from build123d import *

# Parameters (mm, degrees)
BOSS_EXTRUDE1_DEPTH             = 12.7
BOSS_EXTRUDE4_REACH             = 14.7
BOSS_EXTRUDE4_DIRECTION_2_REACH = 14.7
SKETCH6_W                       = 16.51
SKETCH6_H                       = 15.748
CUT_EXTRUDE2_DEPTH              = 53.07
SKETCH11_W                      = 11.43
SKETCH11_H                      = 7.62
CUT_EXTRUDE3_DEPTH              = 3.81
SKETCH15_R                      = 3.2385
CUT_EXTRUDE4_DEPTH              = 25.4


with BuildPart() as part:
    # Sketch1 → Boss-Extrude1 (new body, symmetric)
    with BuildSketch(Plane.XY):
        with BuildLine():
            Line((-20.32, 16.002), (-20.32, -25.4))
            Line((-20.32, -25.4), (20.32, -25.4))
            Line((20.32, -25.4), (20.32, 16.002))
            Line((20.32, 16.002), (2.794, 16.002))
            Line((2.794, 16.002), (2.794, 28.1305))
            Line((2.794, 28.1305), (6.477, 28.1305))
            ThreePointArc((6.477, 28.1305), (6.946330803, 28.444096816), (6.836210245, 28.997710245))
            Line((6.836210245, 28.997710245), (3.706459265, 32.127461224))
            ThreePointArc((3.706459265, 32.127461224), (2.882423959, 32.678064013), (1.910408041, 32.87141))
            Line((1.910408041, 32.87141), (-1.910408041, 32.87141))
            ThreePointArc((-1.910408041, 32.87141), (-2.882423959, 32.678064013), (-3.706459265, 32.127461224))
            Line((-3.706459265, 32.127461224), (-6.836210245, 28.997710245))
            ThreePointArc((-6.836210245, 28.997710245), (-6.946330803, 28.444096816), (-6.477, 28.1305))
            Line((-6.477, 28.1305), (-2.794, 28.1305))
            Line((-2.794, 28.1305), (-2.794, 16.002))
            Line((-2.794, 16.002), (-20.32, 16.002))
        make_face()
        Polygon((-4.106115114, 7.112), (-8.212230229, 0), (-4.106115114, -7.112), (4.106115114, -7.112), (8.212230229, 0), (4.106115114, 7.112), align=None, mode=Mode.SUBTRACT)
    extrude(amount=BOSS_EXTRUDE1_DEPTH, both=True)

    # Boss-Extrude4: up to this face of the body (flat: up to its plane)
    boss_extrude4_end = Plane(part.part.faces().sort_by_distance((-6.289975232, 28.715968196, 12.7))[0])
    # Sketch10 → Boss-Extrude4 (add, up to the picked face)
    with BuildSketch(Plane.XY, mode=Mode.PRIVATE) as boss_extrude4_sk1:
        Polygon((-20.32, -25.4), (-20.32, -46.99), (-31.75, -46.99), (-31.75, -50.8), (-16.51, -50.8), (-16.51, -25.4), align=None)
    boss_extrude4_tool1 = split(extrude(boss_extrude4_sk1.sketch, amount=BOSS_EXTRUDE4_REACH, mode=Mode.PRIVATE), bisect_by=boss_extrude4_end, keep=Keep.BOTH, mode=Mode.PRIVATE)
    add(boss_extrude4_tool1.solids().sort_by_distance((-20.023788, -36.195, 0))[0])

    # Boss-Extrude4 direction 2: up to this face of the body (flat: up to its plane)
    boss_extrude4_direction_2_end = Plane(part.part.faces().sort_by_distance((-6.289975232, 28.715968196, -12.7))[0])
    # Sketch10 → Boss-Extrude4 direction 2 (add, up to the picked face)
    with BuildSketch(Plane.XY, mode=Mode.PRIVATE) as boss_extrude4_direction_2_sk1:
        Polygon((-20.32, -25.4), (-20.32, -46.99), (-31.75, -46.99), (-31.75, -50.8), (-16.51, -50.8), (-16.51, -25.4), align=None)
    boss_extrude4_direction_2_tool1 = split(extrude(boss_extrude4_direction_2_sk1.sketch, amount=-BOSS_EXTRUDE4_DIRECTION_2_REACH, mode=Mode.PRIVATE), bisect_by=boss_extrude4_direction_2_end, keep=Keep.BOTH, mode=Mode.PRIVATE)
    add(boss_extrude4_direction_2_tool1.solids().sort_by_distance((-20.023788, -36.195, 0))[0])

    # Sketch6 → Cut-Extrude2 (cut, through all)
    with BuildSketch(Plane(origin=(20.32, 0, 0), x_dir=(0, 0, -1), z_dir=(1, 0, 0))):
        with Locations((0, -17.526)):
            Rectangle(SKETCH6_W, SKETCH6_H)
    extrude(amount=-CUT_EXTRUDE2_DEPTH, mode=Mode.SUBTRACT)

    # Sketch11 → Cut-Extrude3 (cut)
    with BuildSketch(Plane(origin=(0, -46.99, 0), x_dir=(1, 0, 0), z_dir=(0, 1, 0))):
        with Locations((-26.035, 0)):
            Rectangle(SKETCH11_W, SKETCH11_H)
    extrude(amount=-CUT_EXTRUDE3_DEPTH, mode=Mode.SUBTRACT)

    # Sketch15 → Cut-Extrude4 (cut)
    with BuildSketch(Plane.XY.offset(12.7)):
        with Locations((0, -19.05)):
            Circle(SKETCH15_R)
    extrude(amount=-CUT_EXTRUDE4_DEPTH, mode=Mode.SUBTRACT)


solid = part.part
Design review of the part built by this model. Coordinates are the model's own, in mm. A direction names the side the tool comes from. Round coordinates to 2 decimals unless told otherwise and drop trailing zeros. Order: outer loops, then holes, each group sorted by start corner. A loop starts at its lowest first (then second) coordinate and runs counter-clockwise, first axis right, second up.
1) Consider section D-D (x = 0). State the section outline as (y, z) points (1 decimal).
The answers:
outline: (-25.4, -12.7) - (-22.3, -12.7) - (-22.3, -8.3) - (-25.4, -8.3) - close; (-25.4, 8.3) - (-22.3, 8.3) - (-22.3, 12.7) - (-25.4, 12.7) - close; (-15.8, -12.7) - (-7.1, -12.7) - (-7.1, 12.7) - (-15.8, 12.7) - (-15.8, 8.3) - (-9.7, 8.3) - (-9.7, -8.3) - (-15.8, -8.3) - close; (7.1, -12.7) - (32.9, -12.7) - (32.9, 12.7) - (7.1, 12.7) - close
2) Draft analysis for pull direction X (two halves, no side actions). For faces 6 (the cylindrical face through (-0.7, -22.21, -10.45)), 7 (the flat face through (0, -7.112, 0)), 8 (the flat face through (20.32, 0, 0)), 9 (the flat face through (-31.75, -49, 8)), state which applies: released by +X, released by -X, zero draft, split by the parting line, or undercut.
The answers:
face 6: undercut
face 7: undercut
face 8: released by +X
face 9: released by -X
3) Clearance check with flat-ended pins moving along their axes: pin 1 Ø2.5 at (x, z) = (-23.5, 10.5) entering from +Y; pin 2 Ø4 at (x, z) = (-1, -2.5) entering from -Y; pin 3 Ø1.1 at (x, z) = (-17.5, -0.5) entering from +Y. State where each tip first meets the part, or that it passes through.
The answers:
pin 1: stops at y = -46.99
pin 2: stops at y = -9.65
pin 3: stops at y = 16
4) Consider section C-C (y = -19.05). State the section outline as (x, z) points (1 decimal), plus the area to 3 significant figures.
The answers:
outline: (-20.3, -12.7) - (-3.2, -12.7) - (-3.2, -8.3) - (-20.3, -8.3) - close; (-20.3, 8.3) - (-3.2, 8.3) - (-3.2, 12.7) - (-20.3, 12.7) - close; (3.2, -12.7) - (20.3, -12.7) - (20.3, -8.3) - (3.2, -8.3) - close; (3.2, 8.3) - (20.3, 8.3) - (20.3, 12.7) - (3.2, 12.7) - close
area: 304 mm2
5) Consider section A-A (z = -0.75). State the section outline as (x, y) points, plus the area to 3 significant figures.
The answers:
outline: (-20.32, -50.8) - (-16.51, -50.8) - (-16.51, -25.4) - (-20.32, -25.4) - close; (-20.32, -9.65) - (20.32, -9.65) - (20.32, 16) - (2.79, 16) - (2.79, 28.13) - (6.48, 28.13) arc R0.51 ccw to (6.84, 29) - (3.71, 32.13) arc R2.54 ccw to (1.91, 32.87) - (-1.91, 32.87) arc R2.54 ccw to (-3.71, 32.13) - (-6.84, 29) arc R0.51 ccw to (-6.48, 28.13) - (-2.79, 28.13) - (-2.79, 16) - (-20.32, 16) - close; hole (-8.21, 0) - (-4.11, -7.11) - (4.11, -7.11) - (8.21, 0) - (4.11, 7.11) - (-4.11, 7.11) - close
area: 1,080 mm2
6) Consider section B-B (x = -28). State the section outline as (y, z) points, plus the area to 3 significant figures.
The answers:
outline: (-50.8, -12.7) - (-46.99, -12.7) - (-46.99, -3.81) - (-50.8, -3.81) - close; (-50.8, 3.81) - (-46.99, 3.81) - (-46.99, 12.7) - (-50.8, 12.7) - close
area: 67.7 mm2
7) Machinability: for faces 1 (the flat face through (-26, -46.99, 8)), 2 (the flat face through (6.13, -3.61, 0.18)), 3 (the flat face through (2, -25.4, -10)), 4 (the flat face through (2.794, 22, 0)), 5 (the flat face through (-2.794, 22, 0)), which of the approach directions +Z, -Z, +X, -X, +Y, -Y give a long, thin tool a straight path to every point of the face, cutting with its end or side? Answer none if there is none.
The answers:
face 1: +Z, -Z, -X, +Y
face 2: +Z, -Z
face 3: +Z, -Z, +X, -Y
face 4: +Z, -Z, +X
face 5: +Z, -Z, -X
8) For L1, parallel to Y at x = 0, z = 10.65; L2, parallel to Z at x = -4, y = -16 (3 decimals); L3, parallel to X at y = 26.5, z = -6.75, list the stretches that pass through material, from the lowest coordinate up.
The answers:
L1: y = -25.4 to -22.29, -15.81 to -7.11, 7.11 to 32.87
L2: z = -12.7 to -8.255, 8.255 to 12.7
L3: x = -2.79 to 2.79
